from build123d import *

# Parameters (mm, degrees)
SKETCH_1_W          = 57
SKETCH_1_H          = 29
EXTRUDE_1_DEPTH     = 2
CUT_EXTRUDE_1_DEPTH = 2
SKETCH_3_R          = 1.525
CUT_EXTRUDE_2_DEPTH = 2


with BuildPart() as part:
    # 草图1 → 凸台-拉伸1 (new body)
    with BuildSketch(Plane.XY):
        Rectangle(SKETCH_1_W, SKETCH_1_H)
    extrude(amount=EXTRUDE_1_DEPTH)

    # 草图2 → 切除-拉伸1 (cut)
    with BuildSketch(Plane.XY.offset(2)):
        Polygon((22.5, 14.5), (28.5, 5), (28.5, 14.5), align=None)
        Polygon((28.5, -14.5), (22.5, -14.5), (28.5, -5), align=None)
    cut_extrude_1 = extrude(amount=-CUT_EXTRUDE_1_DEPTH, mode=Mode.SUBTRACT)

    # 镜向1: 切除-拉伸1 across plane
    add(cut_extrude_1.mirror(Plane(origin=(0, 0, 0), x_dir=(0, 0, 1), z_dir=(1, 0, 0))), mode=Mode.SUBTRACT)

    # 草图3 → 切除-拉伸2 (cut)
    with BuildSketch(Plane.XY.offset(2)):
        with Locations((25.362669783, 0)):
            Circle(SKETCH_3_R)
        with Locations(Location((-25.362669783, 0, 0), (0, 0, 180))):
            Circle(SKETCH_3_R)
    extrude(amount=-CUT_EXTRUDE_2_DEPTH, mode=Mode.SUBTRACT)


solid = part.part
The listing builds one solid part. Answer for the finished solid, in the listing's coordinates (mm). Round coordinates to 2 decimals unless told otherwise and drop trailing zeros. Write each loop counter-clockwise with the first axis right and the second up, starting at its lowest first coordinate (ties: lowest second). Pieces come first, ordered by that corner, then holes. Notation, with made-up numbers: (-1, 64.25) - (5, 64.25) arc R13 ccw to (5, 89.25) - close; hole circle Ø10 at (83.25, 29.5). An arc over 180 degrees is marked (long way). Use a Markdown table: item, result. Add a question column.
1. For a pull along Y with two mould halves and no side action, classify faces 1 (the face through (-23.84, -0.07, 1.01)), 2 (the face through (28.5, 0, 1)), 3 (the face through (25.458, -9.816, 1.014)), 4 (the face through (23.84, 0.07, 1.01)) as +Y half, -Y half, draft (parallel to the pull), parting line (faces both ways), or undercut.
2. The part is cut by section D-D (y = 5.75). Write down the section's boundary in (x, z).
3. Consider line 1 (X direction, y = 1, z = 1.6); line 2 (X direction, y = -8.5, z = 1.95); line 3 (X direction, y = 6.25, z = 1.55). Determine where each line is inside the solid, lowest interval first.
4. The part is cut by section A-A (y = 0). Write down the section's boundary in (x, z), and give its area (3 significant figures).
5. The part is cut by section C-C (y = 12.25). Write down the section's boundary in (x, z).
6. The part is cut by section B-B (z = 0.9). Write down the section's boundary in (x, y) (3 decimals), and give its area (3 significant figures).
Reported:
| question | item | result |
|---|---|---|
| 1 | face 1 | undercut |
| 1 | face 2 | draft |
| 1 | face 3 | -Y half |
| 1 | face 4 | undercut |
| 2 | outline | (-28.03, 0) - (28.03, 0) - (28.03, 2) - (-28.03, 2) - close |
| 3 | line 1 | -28.5 to -26.51, -24.21 to 24.21, 26.51 to 28.5 |
| 3 | line 2 | -26.29 to 26.29 |
| 3 | line 3 | -27.71 to 27.71 |
| 4 | outline | (-28.5, 0) - (-26.89, 0) - (-26.89, 2) - (-28.5, 2) - close; (-23.84, 0) - (23.84, 0) - (23.84, 2) - (-23.84, 2) - close; (26.89, 0) - (28.5, 0) - (28.5, 2) - (26.89, 2) - close |
| 4 | area | 102 mm^2 |
| 5 | outline | (-23.92, 0) - (23.92, 0) - (23.92, 2) - (-23.92, 2) - close |
| 6 | outline | (-28.5, -5) - (-22.5, -14.5) - (22.5, -14.5) - (28.5, -5) - (28.5, 5) - (22.5, 14.5) - (-22.5, 14.5) - (-28.5, 5) - close; hole circle Ø3.05 at (-25.363, 0); hole circle Ø3.05 at (25.363, 0) |
| 6 | area | 1,520 mm^2 |
